from build123d import *

# Parameters (mm, degrees)
F1_DEPTH             = 50.8
F3_DEPTH             = 50.8
F6_D                 = 3.7973
F6_CSINK_D           = 10.4394
F6_CSINK_ANGLE       = 82
F6_ON_F5_D           = 3.7973
F6_ON_F5_CSINK_D     = 10.4394
F6_ON_F5_CSINK_ANGLE = 82
F7_SIZE              = 6.35
F9_SIZE              = 5.08


# Not quite as in the source:
# - a feature of the source that left no trace in its solid (it failed there, or was rolled back) is left out
# - a feature names something its author has since deleted; it is built from what else it names


with BuildPart() as f1:
    # F0 (on Top) → F1 (new body)
    with BuildSketch(Plane.XY):
        Polygon((-61.9125, 0), (0, 0), (0, 61.9125), (-11.1125, 61.9125), (-11.1125, 11.1125), (-61.9125, 11.1125), align=None)
    extrude(amount=-F1_DEPTH)

    # F2 (on face) → F3 (join)
    with BuildSketch(Plane.XY):
        Polygon((0, 0), (0, 61.9125), (-9.525, 61.9125), (-9.525, 9.525), (-61.9125, 9.525), (-61.9125, 0), align=None)
    extrude(amount=F3_DEPTH)

    # F6 (through all)
    with Locations(Plane.YZ):
        with Locations((33.3375, -15.875), (33.3375, 15.875)):
            CounterSinkHole(F6_D / 2, F6_CSINK_D / 2, counter_sink_angle=F6_CSINK_ANGLE)

    # F6 on F5 (through all)
    with Locations(Plane.XZ):
        with Locations((-33.3375, 34.925), (-33.3375, -34.925)):
            CounterSinkHole(F6_ON_F5_D / 2, F6_ON_F5_CSINK_D / 2, counter_sink_angle=F6_ON_F5_CSINK_ANGLE)

    # F7
    f7_edges = [f1.edges().sort_by_distance(p)[0] for p in [
        (0, 0, 0),
    ]]
    chamfer(f7_edges, length=F7_SIZE)

    # F9
    f9_edges = [f1.edges().sort_by_distance(p)[0] for p in [
        (-34.13125, 0, 50.8),
        (-3.175, 3.175, 50.8),
        (0, 34.13125, 50.8),
        (-3.175, 3.175, -50.8),
        (-34.13125, 0, -50.8),
        (0, 34.13125, -50.8),
        (-61.9125, 0, 0),
        (0, 61.9125, 0),
    ]]
    chamfer(f9_edges, length=F9_SIZE)


solid = f1.part
Could you check a few things on this model? Use its own coordinates, in mm. A direction names the side the tool comes from. Round coordinates to 2 decimals unless told otherwise and drop trailing zeros. Order: outer loops, then holes, each group sorted by start corner. A loop starts at its lowest first (then second) coordinate and runs counter-clockwise, first axis right, second up. Notation, with made-up numbers: M 72.25,8.5 L 86.25,8.5 A17 cw 86.25,18.5 Z; hole C -3.75,5 d1. An arc over 180 degrees is marked long. One line per item, written item: value.
(1) I'm going to push flat-ended pins straight in: P1, Ø4.5, axis at x = -33.34, z = -34.92, coming from the -Y side; P2, Ø2.5, axis at y = 33.34, z = 15.88, coming from the -X side; P3, Ø1.5, axis at y = 50.5, z = -20, coming from the -X side; P4, Ø6, axis at x = -33.34, z = 34.92, coming from the -Y side. Where does each tip first touch, or does it pass through?
Ans:
P1: stops at y = 3.41
P2: passes through
P3: stops at x = -11.11
P4: stops at y = 2.55
(2) Imagine slicing it at B-B (y = 41). Write out the boundary of the cut face in (x, z) (1 decimal).
Ans:
outline: M -11.1,-50.8 L -5.1,-50.8 L 0,-45.7 L 0,45.7 L -5.1,50.8 L -9.5,50.8 L -9.5,0 L -11.1,0 Z
(3) Imagine slicing it at C-C (z = -7). Write out the boundary of the cut face in (x, y), and give its area (3 significant figures).
Ans:
outline: M -61.91,5.08 L -56.83,0 L -6.35,0 L 0,6.35 L 0,56.83 L -5.08,61.91 L -11.11,61.91 L -11.11,11.11 L -61.91,11.11 Z
area: 1,210 mm^2
(4) Which directions (+Z, -Z, +X, -X, +Y, -Y) give clear straight access to the entire face, cutting with the end or side of a thin tool? Please do faces 1 (the flat face through (-35, 9.525, 25)), 2 (the flat face through (-36, 11.112, -25)), 3 (the flat face through (-23, 8, 50.8)).
Ans:
face 1: +Z, -X, +Y
face 2: +Z, -Z, -X, +Y
face 3: +Z, +X, -X, +Y, -Y
(5) Imagine slicing it at A-A (x = -25.5). Write out the boundary of the cut face in (y, z) (1 decimal).
Ans:
outline: M 0,-45.7 L 5.1,-50.8 L 11.1,-50.8 L 11.1,0 L 9.5,0 L 9.5,50.8 L 5.1,50.8 L 0,45.7 Z
(6) I need wall thicknesses on line 1 along X through (y, z) = (47.5, -4.5); line 2 along Y through (x, z) = (-25, 14) (3 decimals); line 3 along Y through (x, z) = (-15.5, -41.5). Which ranges of each line are inside material? Lowest first, please. Write a range as from..to.
Ans:
line 1: x = -11.11..0
line 2: y = 0..9.525
line 3: y = 0..11.11
(7) If we mould it in two halves opening along Z, with no side actions, what happens to faces 4 (the cylindrical face through (-34.21, 6.71, 33.24)), 5 (the flat face through (0, 31, -1)), 6 (the flat face through (-2.58, 33.74, -48.3))? For each: released by +Z, released by -Z, zero draft, split by the parting line, or undercut.
Ans:
face 4: undercut
face 5: zero draft
face 6: released by -Z
